```python
from build123d import *

# Parameters (mm, degrees)
SKETCH1_R            = 45.974
SKETCH1_R_2          = 27.4955
SKETCH1_R_3          = 6.5
BOSS_EXTRUDE1_DEPTH  = 6.21400078
M8_CLEARANCE_HOLE1_D = 9
CIRPATTERN1_COUNT    = 9
CUT_EXTRUDE1_DEPTH   = 7.21400078
FILLET1_R            = 2.54


with BuildPart() as part:
    # Sketch1 → Boss-Extrude1 (new body)
    with BuildSketch(Plane(origin=(0, 0, 0), x_dir=(1, 0, 0), z_dir=(0, 1, 0))):
        Circle(SKETCH1_R)
        Circle(SKETCH1_R_2, mode=Mode.SUBTRACT)
        with Locations((-13.33878559, 36.648012211)):
            Circle(SKETCH1_R_3, mode=Mode.SUBTRACT)
        with Locations((13.33878559, 36.648012211)):
            Circle(SKETCH1_R_3, mode=Mode.SUBTRACT)
    extrude(amount=BOSS_EXTRUDE1_DEPTH)

    # M8 Clearance Hole1 (through all)
    with Locations(Plane(origin=(0, 6.21400078, 0), x_dir=(1, 0, 0), z_dir=(0, 1, 0))):
        with Locations((0, 39)):
            m8_clearance_hole1 = Hole(M8_CLEARANCE_HOLE1_D / 2)

    # CirPattern1: M8 Clearance Hole1 ×9 about axis
    cirpattern1_axis = Axis((0, 0, 0), (0, 1, 0))
    for i in range(1, CIRPATTERN1_COUNT):
        add(m8_clearance_hole1.rotate(cirpattern1_axis, i * 360 / CIRPATTERN1_COUNT), mode=Mode.SUBTRACT)

    # Sketch6 → Cut-Extrude1 (cut, through all)
    with BuildSketch(Plane(origin=(0, 6.21400078, 0), x_dir=(1, 0, 0), z_dir=(0, 1, 0))):
        with BuildLine():
            Line((17.934979667, 32.051818133), (24.674577095, 38.79141556))
            ThreePointArc((24.674577095, 38.79141556), (16.105864692, 43.06053644), (6.83878559, 45.462508594))
            Line((6.83878559, 45.462508594), (6.83878559, 36.648012211))
            ThreePointArc((6.83878559, 36.648012211), (15.8262279, 42.653229172), (17.934979667, 32.051818133))
        make_face()
        with BuildLine():
            Line((-6.83878559, 36.648012211), (-6.83878559, 45.462508594))
            ThreePointArc((-6.83878559, 45.462508594), (-13.487094864, 43.951188245), (-19.83878559, 41.473259606))
            Line((-19.83878559, 41.473259606), (-19.83878559, 36.648012211))
            ThreePointArc((-19.83878559, 36.648012211), (-13.33878559, 43.148012211), (-6.83878559, 36.648012211))
        make_face()
    extrude(amount=-CUT_EXTRUDE1_DEPTH, mode=Mode.SUBTRACT)

    # Fillet1
    fillet1_edges = [part.edges().sort_by_distance(p)[0] for p in [
        (6.83878559, 3.10700039, -45.462508594),
        (24.674577095, 3.10700039, -38.79141556),
        (-19.83878559, 3.10700039, -41.473259606),
        (-6.83878559, 3.10700039, -45.462508594),
    ]]
    fillet(fillet1_edges, radius=FILLET1_R)


solid = part.part
```
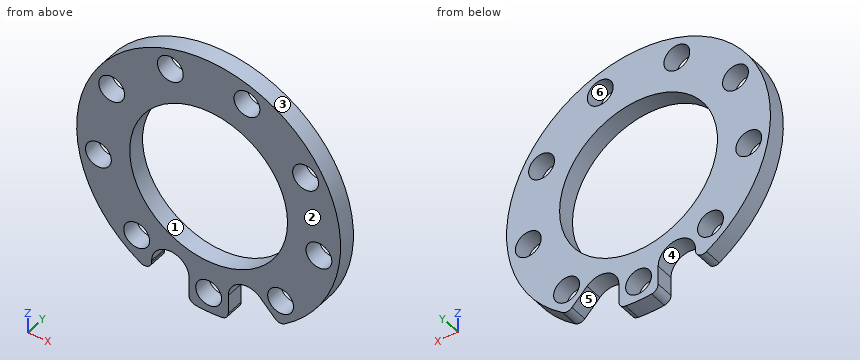
Verification items for the finished model (mm, model axes). Face numbers are marked on the shaded views. A direction names the side the tool comes from. Coordinates: 2 decimals unless noted, no trailing zeros. Loops run counter-clockwise (first coordinate to the right, second up) from the corner with the lowest first, then second, coordinate; pieces in that order, holes last. Notation, with made-up numbers: (82.25, 13) -> (99.25, 13) arc R15 ccw to (99.25, 29) -> close; hole circle Ø11 at (83.5, 53). An arc over 180 degrees is marked (long way). Put each result on its own line as item: value.
1. Thickness scan on line 1 (Z direction, x = 0, y = 4.25); line 2 (Z direction, x = -3, y = 1.5); line 3 (X direction, y = 1.75, z = -37). Record the ranges inside material, lowest first.
Result set:
line 1: z = -45.97 to -43.5, -34.5 to -27.5, 27.5 to 45.97
line 2: z = -45.88 to -42.35, -35.65 to -27.33, 27.33 to 45.88
line 3: x = -27.29 to -19.84, -6.84 to -4.03, 4.03 to 6.84, 22.88 to 27.29
2. Mould release check, pull along Z, two halves, no side actions. Record for the marked faces 1, 2, 3 and 4: pulls with the +Z half, pulls with the -Z half, needs draft (parallel to the pull), parting line crosses it, or undercut.
Result set:
face 1: undercut
face 2: needs draft
face 3: parting line crosses it
face 4: pulls with the -Z half
3. Tool access check on the marked faces 5 and 6. Record the directions out of +Z, -Z, +X, -X, +Y, -Y that give a thin tool (end or side, any length) a straight path to the whole face; none if there is none.
Result set:
face 5: -Z, +Y, -Y
face 6: +Y, -Y
4. Section check A-A, the plane x = 0. Record the boundary of the cut face in (y, z), then the cut area to 3 significant figures.
Result set:
outline: (0, -45.97) -> (6.21, -45.97) -> (6.21, -43.5) -> (0, -43.5) -> close; (0, -34.5) -> (6.21, -34.5) -> (6.21, -27.5) -> (0, -27.5) -> close; (0, 27.5) -> (6.21, 27.5) -> (6.21, 45.97) -> (0, 45.97) -> close
area: 174 mm^2
5. Section check B-B, the plane z = -24. Record the boundary of the cut face in (x, y).
Result set:
outline: (-39.21, 0) -> (-13.42, 0) -> (-13.42, 6.21) -> (-39.21, 6.21) -> close; (13.42, 0) -> (39.21, 0) -> (39.21, 6.21) -> (13.42, 6.21) -> close
6. Gauge pin test, flat ends, axial feed: P1, Ø2, axis at y = 3.5, z = 26, coming from the +X side; P2, Ø2, axis at x = -33, y = 3, coming from the +Z side; P3, Ø0.6, axis at y = 2.5, z = -37, coming from the +X side. Record the tip position at first contact, or that the pin passes through.
Result set:
P1: stops at x = 38.58
P2: stops at z = 33.01
P3: stops at x = 27.69
7. Section check D-D, the plane z = 19.5. Record the boundary of the cut face in (x, y) (3 decimals).
Result set:
outline: (-41.634, 0) -> (-38.275, 0) -> (-38.275, 6.214) -> (-41.634, 6.214) -> close; (-29.275, 0) -> (-19.384, 0) -> (-19.384, 6.214) -> (-29.275, 6.214) -> close; (19.384, 0) -> (29.275, 0) -> (29.275, 6.214) -> (19.384, 6.214) -> close; (38.275, 0) -> (41.634, 0) -> (41.634, 6.214) -> (38.275, 6.214) -> close
8. Section check C-C, the plane y = 5. Give the number of separate pieces and of enclosed holes in the cut face, then the cut area to 3 significant figures.
Result set:
separate pieces: 1
enclosed holes: 10
area: 3,350 mm^2
